For this review, take the finished solid that the model builds, in its own axes (mm). Give positions to 0.01 mm unless a question says otherwise; leave off trailing zeros. Loops run counter-clockwise (first coordinate to the right, second up) from the corner with the lowest first, then second, coordinate; pieces in that order, holes last.
```python
from build123d import *

# Parameters (mm, degrees)
BOSS_EXTRUDE1_DEPTH = 100
FILLET2_R           = 3


with BuildPart() as part:
    # Sketch2 → Boss-Extrude1 (new body)
    with BuildSketch(Plane(origin=(0, 0, 0), x_dir=(1, 0, 0), z_dir=(0, 1, 0))):
        Polygon((0, -47), (-8, -47), (-8, -49.8), (-10, -49.8), (-10, -47.4), (-10, 47.6), (-10, 50), (-8, 50), (-8, 47), (0, 47), align=None)
    extrude(amount=BOSS_EXTRUDE1_DEPTH)

    # Fillet2
    fillet2_edges = [part.edges().sort_by_distance(p)[0] for p in [
        (0, 100, 0),
    ]]
    fillet(fillet2_edges, radius=FILLET2_R)

    # Sketch3 → Cut-Revolve1 (revolve, cut)
    with BuildSketch(Plane.XY):
        with BuildLine():
            Line((-3.5, 85), (11.5, 85))
            ThreePointArc((11.5, 85), (4, 92.5), (-3.5, 85))
        make_face()
    revolve(axis=Axis((-3.5, 85, 0), (1, 0, 0)), mode=Mode.SUBTRACT)


solid = part.part
```
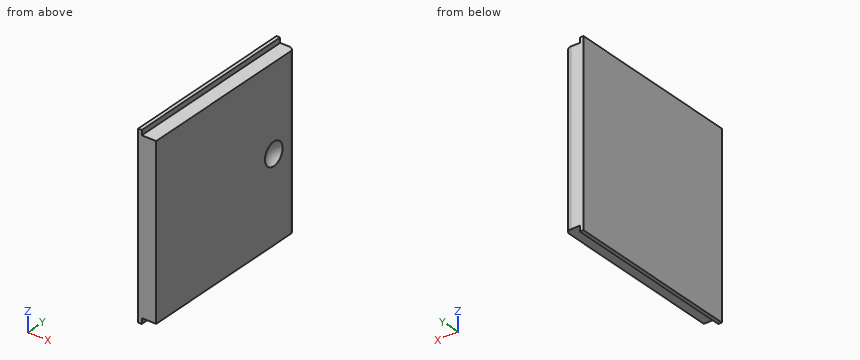
Item 1: Take a section at B-B on x = -5. Give the boundary of the cut face in (y, z), and give its area (3 significant figures).
Answer:
outline: (0, -47) - (100, -47) - (100, 47) - (0, 47) - close
area: 9,400 mm2
Item 2: Take a section at C-C on y = 83.5. Give the boundary of the cut face in (x, z).
Answer:
outline: (-10, -50) - (-8, -50) - (-8, -47) - (0, -47) - (0, -6.16) arc R7.35 cw to (0, 6.16) - (0, 47) - (-8, 47) - (-8, 49.8) - (-10, 49.8) - close
Item 3: For L1, parallel to Z at x = -4.25, y = 78; L2, parallel to Y at x = -2.75, z = -6; L3, parallel to Y at x = -1.5, z = 2.5, list the stretches that pass through material, from the lowest coordinate up.
Answer:
L1: z = -47 to 47
L2: y = 0 to 99.99
L3: y = 0 to 80.56, 89.44 to 99.6
Item 4: Take a section at A-A on y = 41. Give the boundary of the cut face in (x, z).
Answer:
outline: (-10, -50) - (-8, -50) - (-8, -47) - (0, -47) - (0, 47) - (-8, 47) - (-8, 49.8) - (-10, 49.8) - close
Item 5: Clearance check with flat-ended pins moving along their axes: pin 1 Ø3 at (y, z) = (47, 49) entering from +X; pin 2 Ø4 at (x, y) = (-3.5, 66) entering from +Z. State where each tip first meets the part, or that it passes through.
Answer:
pin 1: stops at x = -8
pin 2: stops at z = 47
